Verification items for the finished model (mm, model axes). A direction names the side the tool comes from. Round coordinates to 2 decimals unless told otherwise and drop trailing zeros. Write each loop counter-clockwise with the first axis right and the second up, starting at its lowest first coordinate (ties: lowest second). Pieces come first, ordered by that corner, then holes. Notation, with made-up numbers: M 86.5,85.25 L 96.5,85.25 A20 ccw 96.5,111.25 Z; hole C 10,-35.75 d7. An arc over 180 degrees is marked long. Answer in a Markdown table with one row per item. Add a question column.
1. Sectioned sample at C-C on z = 154.5. Record the cut outline in (x, y).
2. Set-up check for faces 1 (the flat face through (1, 0, 100)), 2 (the flat face through (34.055, -78.88, -47.456)): record each of +Z, -Z, +X, -X, +Y, -Y from which the full face is reachable in a straight line by a thin tool's end or side.
3. Material ranges on probe 1 along X at (y, z) = (-95, 102.5); probe 2 along Z at (x, y) = (13.5, -14.5); probe 3 along Z at (x, y) = (5, -44), recorded low to high.
4. Sectioned sample at A-A on y = -49. Record the cut outline in (x, z).
5. Draft check along Z on faces 3 (the flat face through (0, -79, 137)), 4 (the flat face through (1.5, -79, 133)), 5 (the flat face through (31.62, -78.88, -46.54)), 6 (the flat face through (11.1, -78.9, 281.8)). Enter one of: pulls with the +Z half, pulls with the -Z half, needs draft (parallel to the pull), parting line crosses it, or undercut.
6. Sectioned sample at D-D on y = -15.5. Record the cut outline in (x, z), plus the area to 3 significant figures.
7. Go/stop test with flat-tipped pins: pin 1 Ø6 at (y, z) = (-116, 99.5) entering from +X; pin 2 Ø4 at (x, y) = (37.5, -34) entering from -Z; pin 3 Ø1.6 at (x, y) = (1, -15) entering from +Z. Record where each tip stops, or that it passes through.
8. Sectioned sample at B-B on z = 230. Record the cut outline in (x, y).
```python
from build123d import *

# Parameters (mm, degrees)
F1_DEPTH = 160
F2_W     = 20
F2_H     = 44
F3_DEPTH = 65.375966


with BuildPart() as f1:
    # F0 (on Front) → F1 (new body)
    with BuildSketch(Plane.XZ):
        with BuildLine():
            Line((0, 270), (0, 0))
            Line((0, 0), (64.134226, -94.399233))
            Line((64.134226, -94.399233), (65.374966, -93.556283))
            Line((65.374966, -93.556283), (1.845681, -0.047463))
            ThreePointArc((1.845681, -0.047463), (1.588373, 0.488525), (1.5, 1.076471))
            Line((1.5, 1.076471), (1.5, 269.405426))
            Line((1.5, 269.405426), (23.016468, 292.282105))
            Line((23.016468, 292.282105), (21.923822, 293.309784))
            Line((21.923822, 293.309784), (0, 270))
        make_face()
    extrude(amount=F1_DEPTH)

    # F2 (on face) → F3 (cut, through all)
    with BuildSketch(Plane(origin=(0, 0, 0), x_dir=(0, -1, 0), z_dir=(-1, 0, 0))):
        with Locations((19, 215)):
            Rectangle(F2_W, F2_H)
        with Locations((47, 215)):
            Rectangle(F2_W, F2_H)
        with Locations((75, 215)):
            Rectangle(F2_W, F2_H)
        with Locations((103, 215)):
            Rectangle(F2_W, F2_H)
        with Locations((19, 153)):
            Rectangle(F2_W, F2_H)
    extrude(amount=-F3_DEPTH, mode=Mode.SUBTRACT)


solid = f1.part
```
Geometry check:
| question | item | result |
|---|---|---|
| 1 | outline | M 0,-160 L 1.5,-160 L 1.5,-29 L 0,-29 Z; M 0,-9 L 1.5,-9 L 1.5,0 L 0,0 Z |
| 2 | face 1 | +Z, -Z, +X, -X, +Y |
| 2 | face 2 | +X, +Y, -Y |
| 3 | probe 1 | x = 0 to 1.5 |
| 3 | probe 2 | z = -19.87 to -17.2, 282.16 to 284.35 |
| 3 | probe 3 | z = -7.36 to -4.69, 273.13 to 275.32 |
| 4 | outline | M 0,0 L 64.13,-94.4 L 65.37,-93.56 L 1.85,-0.05 A2 cw 1.5,1.08 L 1.5,193 L 0,193 Z; M 0,237 L 1.5,237 L 1.5,269.41 L 23.02,292.28 L 21.92,293.31 L 0,270 Z |
| 5 | face 3 | needs draft |
| 5 | face 4 | undercut |
| 5 | face 5 | pulls with the -Z half |
| 5 | face 6 | pulls with the +Z half |
| 6 | outline | M 0,0 L 64.13,-94.4 L 65.37,-93.56 L 1.85,-0.05 A2 cw 1.5,1.08 L 1.5,131 L 0,131 Z; M 0,175 L 1.5,175 L 1.5,193 L 0,193 Z; M 0,237 L 1.5,237 L 1.5,269.41 L 23.02,292.28 L 21.92,293.31 L 0,270 Z |
| 6 | area | 491 mm2 |
| 7 | pin 1 | stops at x = 1.5 |
| 7 | pin 2 | stops at z = -58.14 |
| 7 | pin 3 | stops at z = 271.91 |
| 8 | outline | M 0,-160 L 1.5,-160 L 1.5,-113 L 0,-113 Z; M 0,-93 L 1.5,-93 L 1.5,-85 L 0,-85 Z; M 0,-65 L 1.5,-65 L 1.5,-57 L 0,-57 Z; M 0,-37 L 1.5,-37 L 1.5,-29 L 0,-29 Z; M 0,-9 L 1.5,-9 L 1.5,0 L 0,0 Z |
